Source: CAD feature listing. Evaluate the final solid. Frame: model axes, mm. A direction names the side the tool comes from. Round coordinates to 2 decimals unless told otherwise and drop trailing zeros. Loops run counter-clockwise (first coordinate to the right, second up) from the corner with the lowest first, then second, coordinate; pieces in that order, holes last. Notation, with made-up numbers: M -12.75,89.5 L 33.25,89.5 A13 ccw 33.25,107.5 Z; hole C -7,18 d7. An arc over 180 degrees is marked long. Write each question's results on one line, items separated by ' | '. Start each with the question number.
1. Ray query, line 1 (X direction, y = 3.65, z = -16.75); line 2 (Z direction, x = 30, y = 5.9); line 3 (Z direction, x = 31, y = 3.9). Return the intervals inside material, ascending.
2. Section C-C on z = -19.5. Output: boundary loops of the cut face in (x, y), and give its area (3 significant figures).
3. Draft query along X for faces 1 (the flat face through (26, 4, -9)), 2 (the flat face through (30.513, 4.465, -19.339)), 3 (the flat face through (31, 5, 0)). Return one class per face: released by +X, released by -X, zero draft, split by the parting line, or undercut.
4. Set-up query: faces 4 (the flat face through (31, 2, -11)), 5 (the flat face through (26.617, 4.535, -17.359)). Return all of +Z, -Z, +X, -X, +Y, -Y with unobstructed straight access to the full face (end or side cutting, diameter ignored); none if empty.
5. Section B-B on x = 30.5. Output: boundary loops of the cut face in (y, z), and give its area (3 significant figures).
6. Section A-A on y = 4.85. Output: boundary loops of the cut face in (x, z).
from build123d import *

# Parameters (mm, degrees)
BOX020_W               = 5
BOX020_H               = 96
BOX020_DEPTH           = 60
BOX020_PLACEMENT_ANGLE = 310
BOX017_W               = 11
BOX017_H               = 5
BOX017_DEPTH           = 22


with BuildPart() as cube020:
    # Box020 → Box020 (new body)
    with BuildSketch(Plane.XY):
        with Locations((2.5, 48)):
            Rectangle(BOX020_W, BOX020_H)
    extrude(amount=BOX020_DEPTH)


with BuildPart() as cube020_1:
    # Box020 placement: moved
    add(cube020.part.moved(Location((70, 2, -59))).rotate(Axis((70, 2, -59), (0, 1, 0)), BOX020_PLACEMENT_ANGLE))


with BuildPart() as cut011:
    # Box017 → Box017 (new body)
    with BuildSketch(Plane(origin=(26, 2, -22), x_dir=(1, 0, 0), z_dir=(0, 0, 1))):
        with Locations((5.5, 2.5)):
            Rectangle(BOX017_W, BOX017_H)
    extrude(amount=BOX017_DEPTH)

    # Cut011: cut Cube020
    add(cube020_1.part, mode=Mode.SUBTRACT)


solid = cut011.part
Taken from the geometry:
1) line 1: 26 to 27.13, 27.43 to 37 | line 2: -18.91 to 0 | line 3: -19.75 to 0
2) outline: M 30.7,2 L 37,2 L 37,7 L 30.7,7 Z | area: 31.5 mm^2
3) face 1: released by -X | face 2: undercut | face 3: zero draft
4) face 4: +Z, -Z, +X, -X, -Y | face 5: -Z, +Y, -Y
5) outline: M 2,-19.33 L 7,-19.33 L 7,0 L 2,0 Z | area: 96.6 mm^2
6) outline: M 26,-18.09 L 27.25,-16.6 L 33.68,-22 L 37,-22 L 37,0 L 26,0 Z
